Verification items for this drawing (mm, ordinates from the low corner). Give positions to 0.01 mm unless a question says otherwise; leave off trailing zeros. Loops run counter-clockwise (first coordinate to the right, second up) from the corner with the lowest first, then second, coordinate; pieces in that order, holes last. Notation, with made-up numbers: M -12,74 L 6,74 A19 cw 6,102 Z; hole C -2.5,24.25 d10. An arc over 180 degrees is marked long. Use one line per item in the form item = value.
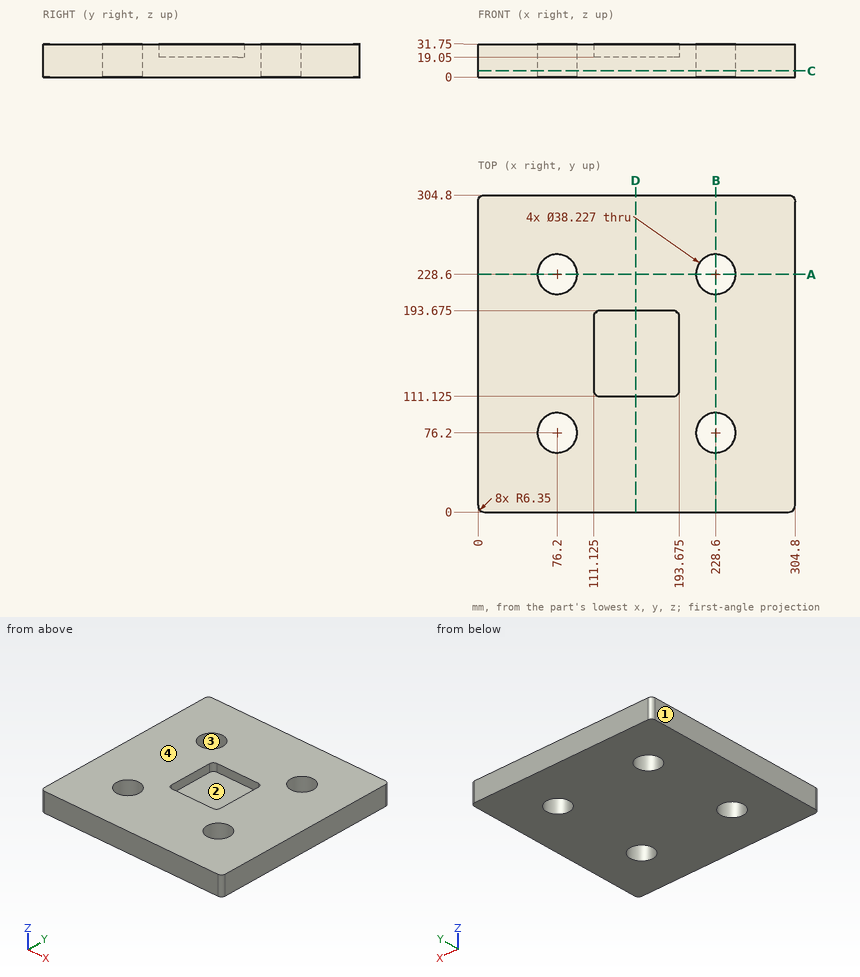
1) Scan lines: line 1 (X direction, y = 228, z = 13); line 2 (Y direction, x = 76.2, z = 9.5); line 3 (X direction, y = 88, z = 29). Record each from-to range of solid material in increasing order.
Evaluation:
line_1 = 0 to 57.1, 95.3 to 209.5, 247.7 to 304.8
line_2 = 0 to 57.09, 95.31 to 209.49, 247.71 to 304.8
line_3 = 0 to 61.16, 91.24 to 213.56, 243.64 to 304.8
2) Section check A-A (y = 228.6). Record the cut outline in (x, z), then the cut area to 3 significant figures.
Evaluation:
outline = M 0,0 L 57.09,0 L 57.09,31.75 L 0,31.75 Z; M 95.31,0 L 209.49,0 L 209.49,31.75 L 95.31,31.75 Z; M 247.71,0 L 304.8,0 L 304.8,31.75 L 247.71,31.75 Z
area = 7,250 mm^2
3) Release check for a two-part mould opening along X. For the marked faces 1, 2, 3 and 4 record: pulls with the +X half, pulls with the -X half, needs draft (parallel to the pull), parting line crosses it, or undercut.
Evaluation:
face_1 = pulls with the -X half
face_2 = undercut
face_3 = undercut
face_4 = needs draft
4) Section check C-C (z = 6). Record the cut outline in (x, y).
Evaluation:
outline = M 0,6.35 A6.35 ccw 6.35,0 L 298.45,0 A6.35 ccw 304.8,6.35 L 304.8,298.45 A6.35 ccw 298.45,304.8 L 6.35,304.8 A6.35 ccw 0,298.45 Z; hole C 76.2,76.2 d38.23; hole C 76.2,228.6 d38.23; hole C 228.6,76.2 d38.23; hole C 228.6,228.6 d38.23
5) Depth check by flat-ended pin: pin 1 Ø25 at (x, y) = (165.5, 161) entering from +Z. Enter the tip coordinate at first touch or a pass-through.
Evaluation:
pin_1 = 19.05
6) Section check D-D (x = 151.5). Record the cut outline in (y, z) (3 decimals).
Evaluation:
outline = M 0,0 L 304.8,0 L 304.8,31.75 L 193.675,31.75 L 193.675,19.05 L 111.125,19.05 L 111.125,31.75 L 0,31.75 Z
